Here's how the part is built. I have some questions about the finished solid (model axes, mm). A direction names the side the tool comes from. Give positions to 0.01 mm unless a question says otherwise; leave off trailing zeros. Loops run counter-clockwise (first coordinate to the right, second up) from the corner with the lowest first, then second, coordinate; pieces in that order, holes last.
Q1. I'm going to push flat-ended pins straight in: P1, Ø12, axis at y = 56, z = -57.5, coming from the -X side; P2, Ø9, axis at y = 162, z = 40.5, coming from the +X side; P3, Ø6, axis at x = 0, y = 100.5, coming from the -Z side. Where does each tip first touch, or does it pass through?
Q2. Suppose I cut it at A-A (x = 0). List the corners of the cut face in (y, z) for me.
Q3. Suppose I cut it at D-D (x = 32). List the corners of the cut face in (y, z) for me.
Q4. Thinking about a two-plate mould opening in Y: for faces 1 (the face through (-13.02, 147.46, -99.15)), 2 (the face through (-1, 0, -1)), 3 (the face through (-55.55, 99.79, -42.594)), 4 (the face through (-1, 200, -1)), which applies, pulls with the +Y half, pulls with the -Y half, needs draft (parallel to the pull), parting line crosses it, or undercut?
Q5. For faces 5 (the face through (68, 85, -21)), 6 (the face through (-50, 165, 1)), 7 (the face through (95.38, 41.9, -30.04)), which set-ups out of +Z, -Z, +X, -X, +Y, -Y let a thin tool reach every point of the face, with its end or its side?
Q6. Suppose I cut it at C-C (z = 0). List the corners of the cut face in (x, y) for me, and give its area (3 significant figures).
Q7. Suppose I cut it at B-B (z = 81). List the corners of the cut face in (x, y) for me.
Q8. I need wall thicknesses on probe 1 along Y at (x, z) = (37.5, 68); probe 2 along Y at (x, z) = (56, -48); probe 3 along Y at (x, z) = (-30, -29.5). Which ranges of each line are inside material? Lowest first, please.
```python
from build123d import *

# Parameters (mm, degrees)
SKETCH2_R               = 100
BOSS_EXTRUDE1_DEPTH     = 200
CUT_EXTRUDE1_DEPTH      = 200
CUT_EXTRUDE1_DEPTH_BACK = 200


with BuildPart() as part:
    # Sketch2 → Boss-Extrude1 (new body)
    with BuildSketch(Plane(origin=(0, 0, 0), x_dir=(1, 0, 0), z_dir=(0, 1, 0))):
        Circle(SKETCH2_R)
    extrude(amount=BOSS_EXTRUDE1_DEPTH)

    # Sketch3 → Cut-Revolve3 (revolve, cut)
    with BuildSketch(Plane.XY):
        Polygon((100, 85), (100, 100), (100, 115), (70, 115), (70, 85), align=None)
    revolve(axis=Axis((0, 235.170477907, 0), (0, -1, 0)), mode=Mode.SUBTRACT)

    # Sketch4 → Cut-Extrude1 (cut, two sides)
    with BuildSketch(Plane.XY) as cut_extrude1_sk:
        Polygon((0, 180), (50, 180), (50, 150), (-50, 150), (-50, 180), align=None)
    extrude(amount=CUT_EXTRUDE1_DEPTH, mode=Mode.SUBTRACT)
    extrude(cut_extrude1_sk.sketch, amount=-CUT_EXTRUDE1_DEPTH_BACK, mode=Mode.SUBTRACT)


solid = part.part
```
Solutions:
1. P1: stops at x = -85.72
1. P2: stops at x = 93.3
1. P3: stops at z = -70
2. outline: (0, -100) - (85, -100) - (85, -70) - (115, -70) - (115, -100) - (150, -100) - (150, 100) - (115, 100) - (115, 70) - (85, 70) - (85, 100) - (0, 100) - close; (180, -100) - (200, -100) - (200, 100) - (180, 100) - close
3. outline: (0, -94.74) - (85, -94.74) - (85, -62.26) - (115, -62.26) - (115, -94.74) - (150, -94.74) - (150, 94.74) - (115, 94.74) - (115, 62.26) - (85, 62.26) - (85, 94.74) - (0, 94.74) - close; (180, -94.74) - (200, -94.74) - (200, 94.74) - (180, 94.74) - close
4. face 1: needs draft
4. face 2: pulls with the -Y half
4. face 3: undercut
4. face 4: pulls with the +Y half
5. face 5: none
5. face 6: +Z, -Z
5. face 7: +Y, -Y
6. outline: (-100, 0) - (100, 0) - (100, 85) - (70, 85) - (70, 115) - (100, 115) - (100, 200) - (-100, 200) - (-100, 115) - (-70, 115) - (-70, 85) - (-100, 85) - close; hole (-50, 150) - (50, 150) - (50, 180) - (-50, 180) - close
6. area: 35,200 mm2
7. outline: (-58.64, 0) - (58.64, 0) - (58.64, 85) - (-58.64, 85) - close; (-58.64, 115) - (58.64, 115) - (58.64, 200) - (-58.64, 200) - close; hole (-50, 150) - (50, 150) - (50, 180) - (-50, 180) - close
8. probe 1: y = 0 to 85, 115 to 150, 180 to 200
8. probe 2: y = 0 to 85, 115 to 200
8. probe 3: y = 0 to 150, 180 to 200
